from build123d import *

# Parameters (mm, degrees)
SKETCH_R         = 6.5
EXTRUDE_DEPTH    = 7.5
TUBE002_R        = 6.5
TUBE002_R_2      = 5
TUBE002_DEPTH    = 2.5
SKETCH023_R      = 1.5
EXTRUDE015_DEPTH = 100
EXTRUDE008_DEPTH = 6.5


with BuildPart() as extrude_body:
    # Sketch (on Tube) → Extrude (new body)
    with BuildSketch(Plane.YZ):
        with BuildLine():
            ThreePointArc((10, 0), (0, 10), (-10, 0))
            Line((-10, 0), (-10, -10))
            Line((-15, -15), (-10, -10))
            Line((-15, -15), (15, -15))
            Line((15, -15), (10, -10))
            Line((10, 0), (10, -10))
        make_face()
        Circle(SKETCH_R, mode=Mode.SUBTRACT)
    extrude(amount=EXTRUDE_DEPTH)


with BuildPart() as extrude_body_1:
    # Extrude placement: moved
    add(extrude_body.part.moved(Location((15, 0, 0))))


with BuildPart() as fusion002:
    # Tube002 → Tube002 (new body)
    with BuildSketch(Plane(origin=(20, 0, 0), x_dir=(0, 0, -1), z_dir=(1, 0, 0))):
        Circle(TUBE002_R)
        Circle(TUBE002_R_2, mode=Mode.SUBTRACT)
    extrude(amount=TUBE002_DEPTH)

    # Fusion002: union Extrude body
    add(extrude_body_1.part)


with BuildPart() as extrude015:
    # Sketch023 → Extrude015 (new body)
    with BuildSketch(Plane.YZ.offset(34.5)):
        with Locations((-7, -18.25)):
            Circle(SKETCH023_R)
        with Locations((7, -18.25)):
            Circle(SKETCH023_R)
    extrude(amount=-EXTRUDE015_DEPTH)


with BuildPart() as extrude008:
    # Sketch015 (on Face7 of Fusion001) → Extrude008 (new body)
    with BuildSketch(Plane(origin=(0, 0, -15), x_dir=(1, 0, 0), z_dir=(0, 0, -1))):
        Polygon((-22.5, 20.399377), (-22.5, -20.399377), (-19.5, -22.5), (-15, -22.5), (-15, 22.5), (-19.5, 22.5), align=None)
    extrude(amount=EXTRUDE008_DEPTH)


with BuildPart() as fusion006:
    # Part__Mirroring: instance of Extrude008
    add(extrude008.part.mirror(Plane(origin=(0, 0, 0), x_dir=(0, -1, 0), z_dir=(1, 0, 0))))

    # Cut004: cut Extrude015
    add(extrude015.part, mode=Mode.SUBTRACT)

    # Fusion006: union Fusion002
    add(fusion002.part)


solid = fusion006.part
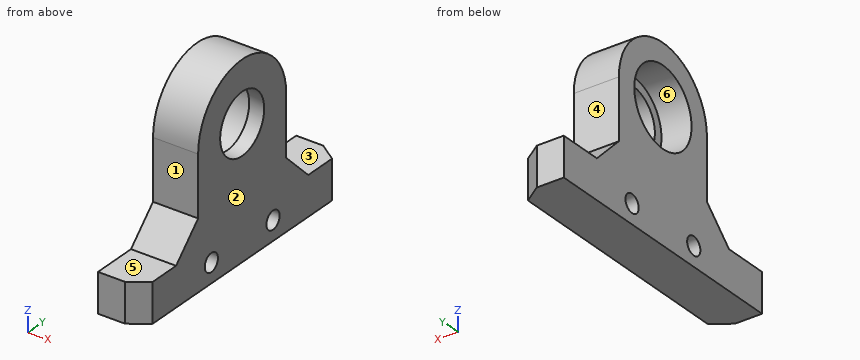
CAD build for the part. Positions are in the model's coordinates, mm. Face numbers are marked on the shaded views. A direction names the side the tool comes from. Round coordinates to 2 decimals unless told otherwise and drop trailing zeros. Order: outer loops, then holes, each group sorted by start corner. A loop starts at its lowest first (then second) coordinate and runs counter-clockwise, first axis right, second up. Notation, with made-up numbers: (-22, 24.5) - (23, 24.5) arc R32 ccw to (23, 58.5) - close; hole circle Ø4 at (-26, 19.5). An arc over 180 degrees is marked (long way). Return JSON: item names as keys, results as strings.
(1) Cut at B-B (y = 0). Give the cut face in (x, z).
Answer key:
{"outline": "(15, -21.5) - (22.5, -21.5) - (22.5, -5) - (20, -5) - (20, -6.5) - (15, -6.5) - close; (15, 6.5) - (20, 6.5) - (20, 5) - (22.5, 5) - (22.5, 10) - (15, 10) - close"}
(2) Cut at A-A (z = -18.25). Give the cut face in (x, y), then the cut area to 3 significant figures.
Answer key:
{"outline": "(15, -22.5) - (19.5, -22.5) - (22.5, -20.4) - (22.5, -8.5) - (15, -8.5) - close; (15, -5.5) - (22.5, -5.5) - (22.5, 5.5) - (15, 5.5) - close; (15, 8.5) - (22.5, 8.5) - (22.5, 20.4) - (19.5, 22.5) - (15, 22.5) - close", "area": "286 mm^2"}
(3) Cut at D-D (z = 2). Give the cut face in (x, y), then the cut area to 3 significant figures.
Answer key:
{"outline": "(15, -9.8) - (22.5, -9.8) - (22.5, -4.58) - (20, -4.58) - (20, -6.18) - (15, -6.18) - close; (15, 6.18) - (20, 6.18) - (20, 4.58) - (22.5, 4.58) - (22.5, 9.8) - (15, 9.8) - close", "area": "62.2 mm^2"}
(4) Pull direction Z, two halves, no side cores. Call the marked faces 4, 5 and 6: +Z half, -Z half, draft (parallel to the pull), parting line (faces both ways), or undercut.
Answer key:
{"face 4": "draft", "face 5": "+Z half", "face 6": "undercut"}
(5) Pin check, flat tips, straight feed: pin 1 Ø1 at (x, z) = (21, 2) entering from +Y; pin 2 Ø5 at (y, z) = (-10.5, -7.5) entering from -X; pin 3 Ø4 at (x, z) = (16, -5.5) entering from -Y; pin 4 Ø4 at (x, y) = (17, 13.5) entering from +Z. Stop position of each tip, or through.
Answer key:
{"pin 1": "stops at y = 9.89", "pin 2": "stops at x = 15", "pin 3": "stops at y = -10", "pin 4": "stops at z = -11.5"}
(6) Tool access for the marked faces 1, 2 and 3: list every direction of +Z, -Z, +X, -X, +Y, -Y with a clear straight run to the whole face (end or side of a thin tool).
Answer key:
{"face 1": "+Z, +X, -X, -Y", "face 2": "+Z, -Z, +X, +Y, -Y", "face 3": "+Z, +X, -X, +Y"}
(7) Cut at C-C (x = 17.5). Give the cut face in (y, z), then the cut area to 3 significant figures.
Answer key:
{"outline": "(-22.5, -21.5) - (22.5, -21.5) - (22.5, -15) - (15, -15) - (10, -10) - (10, 0) arc R10 ccw to (-10, 0) - (-10, -10) - (-15, -15) - (-22.5, -15) - close; hole circle Ø3 at (-7, -18.25); hole circle Ø13 at (0, 0); hole circle Ø3 at (7, -18.25)", "area": "628 mm^2"}
(8) Wall check: probe 1 along Z at (x, y) = (16.9, 0); probe 2 along Y at (x, z) = (22, -7.5); probe 3 along Y at (x, z) = (22, 3). Give the ranges that are in metal, low to high. Write a range as from..to.
Answer key:
{"probe 1": "z = -21.5..-6.5, 6.5..10", "probe 2": "y = -10..10", "probe 3": "y = -9.54..-4, 4..9.54"}
